The model under review builds one solid part; all positions refer to its coordinate system, in mm. Face numbers are marked on the shaded views. A direction names the side the tool comes from. Coordinates: 2 decimals unless noted, no trailing zeros. Order: outer loops, then holes, each group sorted by start corner. A loop starts at its lowest first (then second) coordinate and runs counter-clockwise, first axis right, second up. Notation, with made-up numbers: (-3, 67) -> (13, 67) arc R25 ccw to (13, 98) -> close; hole circle Ø6 at (53.5, 40). An arc over 180 degrees is marked (long way). Put each result on its own line as item: value.
Autodesk Inventor part; units mm, degrees
ref_plane "YZ Plane" through (0, 0, 0) normal (1, 0, 0) x (0, 1, 0)
ref_plane "XZ Plane" through (0, 0, 0) normal (0, 1, 0) x (-1, 0, 0)
ref_plane "XY Plane" through (0, 0, 0) normal (0, 0, 1) x (1, 0, 0)
sketch "Sketch1" plane through (0, 0, 0) normal (0, 0, 1) x (1, 0, 0)
  line L0 (0, 0) -> (85.725, 0)
  line L1 (0, 0) -> (85.725, 0) construction
  line L2 (85.725, 0) -> (85.725, 50.8)
  line L3 (85.725, 50.8) -> (82.55, 50.8)
  line L4 (82.55, 50.8) -> (82.55, 3.175)
  line L5 (82.55, 3.175) -> (3.175, 3.175)
  line L6 (3.175, 3.175) -> (3.175, 28.575)
  line L7 (3.175, 28.575) -> (0, 28.575)
  line L8 (0, 28.575) -> (0, 0)
  dimension "d0" = 85.725
  dimension "d1" = 0
  dimension "d2" = 50.8
  dimension "d3" = 90
  dimension "d4" = 3.175
  dimension "d5" = 47.625
  dimension "d6" = 79.375
  dimension "d7" = 25.4
extrude "Extrusion1" add sketch "Sketch1" along normal blind 584.2
properties part number "FrameFandB"
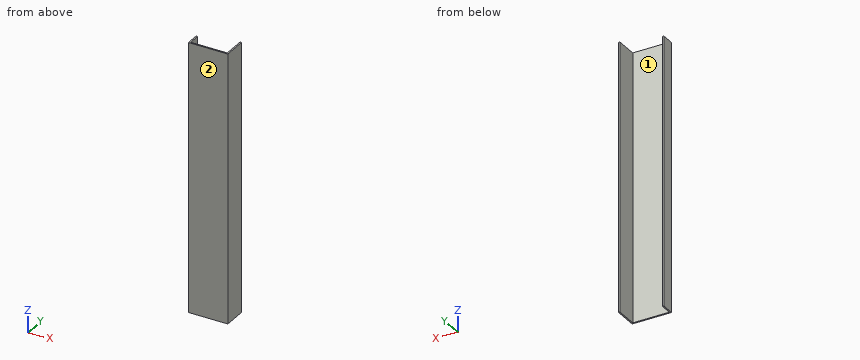
Item 1: Consider section B-B on z = 367.5. Write out the cut boundary in (x, y) (3 decimals), and give its area (3 significant figures).
Answers below:
outline: (0, 0) -> (85.725, 0) -> (85.725, 50.8) -> (82.55, 50.8) -> (82.55, 3.175) -> (3.175, 3.175) -> (3.175, 28.575) -> (0, 28.575) -> close
area: 504 mm^2
Item 2: For the marked faces 1 and 2, list the 3-axis set-ups (+Z, -Z, +X, -X, +Y, -Y) from which the entire face can be reached by the end or side of a thin tool; tool diameter is ignored.
Answers below:
face 1: +Z, -Z, +Y
face 2: +Z, -Z, +X, -X, -Y
Item 3: Consider section C-C on x = 53.5. Write out the cut boundary in (y, z) (3 decimals), and give its area (3 significant figures).
Answers below:
outline: (0, 0) -> (3.175, 0) -> (3.175, 584.2) -> (0, 584.2) -> close
area: 1,850 mm^2
Item 4: For pin 1 Ø14.5 at (y, z) = (32.5, 191.5) entering from -X; pin 2 Ø6 at (x, y) = (27, 8) entering from -Z; pin 3 Ø8 at (x, z) = (24.5, 358.5) entering from +Y (3 decimals); pin 4 Ø1.6 at (x, z) = (2.5, 299.5) entering from +Y (3 decimals), all flat-tipped, find the tip position at first contact; note any pin that passes through.
Answers below:
pin 1: x = 0
pin 2: through
pin 3: y = 3.175
pin 4: y = 28.575
Item 5: Consider section D-D on y = 46. Write out the cut boundary in (x, z) (3 decimals), and give its area (3 significant figures).
Answers below:
outline: (82.55, 0) -> (85.725, 0) -> (85.725, 584.2) -> (82.55, 584.2) -> close
area: 1,850 mm^2
Item 6: For line 1 (X direction, y = 23.5, z = 92.5) (3 decimals); line 2 (Y direction, x = 80.5, z = 497) (3 decimals); line 3 (X direction, y = 32, z = 289.5) (3 decimals), list the stretches that pass through material, from the lowest coordinate up. Write a range as from..to.
Answers below:
line 1: 0..3.175, 82.55..85.725
line 2: 0..3.175
line 3: 82.55..85.725
Item 7: Consider section A-A on y = 13.5. Write out the cut boundary in (x, z) (3 decimals), and give its area (3 significant figures).
Answers below:
outline: (0, 0) -> (3.175, 0) -> (3.175, 584.2) -> (0, 584.2) -> close; (82.55, 0) -> (85.725, 0) -> (85.725, 584.2) -> (82.55, 584.2) -> close
area: 3,710 mm^2
